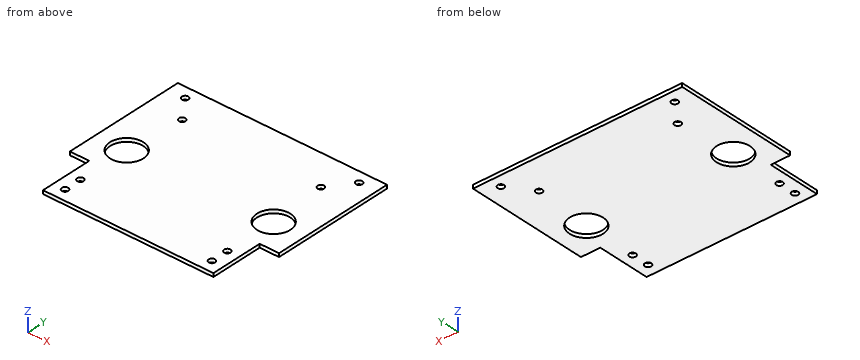
from build123d import *

# Parameters (mm, degrees)
SKETCH1_W           = 178.16
SKETCH1_H           = 150
BOSS_EXTRUDE1_DEPTH = 3
SKETCH2_R           = 14.225
SKETCH2_R_2         = 2.75
CUT_EXTRUDE1_DEPTH  = 4
SKETCH4_W           = 16.5
SKETCH4_H           = 45
CUT_EXTRUDE3_DEPTH  = 4
SKETCH5_R           = 2.75
CUT_EXTRUDE4_DEPTH  = 4


with BuildPart() as part:
    # Sketch1 → Boss-Extrude1 (new body)
    with BuildSketch(Plane.XY):
        with Locations((89.08, -75)):
            Rectangle(SKETCH1_W, SKETCH1_H)
    extrude(amount=BOSS_EXTRUDE1_DEPTH)

    # Sketch2 → Cut-Extrude1 (cut, through all)
    with BuildSketch(Plane.XY.offset(3)):
        with Locations((26.5, -80)):
            Circle(SKETCH2_R)
        with Locations((151.66, -80)):
            Circle(SKETCH2_R)
        with Locations((26.5, -140)):
            Circle(SKETCH2_R_2)
        with Locations((151.66, -140)):
            Circle(SKETCH2_R_2)
        with Locations((26.5, -125)):
            Circle(SKETCH2_R_2)
        with Locations((151.66, -125)):
            Circle(SKETCH2_R_2)
    extrude(amount=-CUT_EXTRUDE1_DEPTH, mode=Mode.SUBTRACT)

    # Sketch4 → Cut-Extrude3 (cut, through all)
    with BuildSketch(Plane.XY.offset(3)):
        with Locations((8.25, -127.5)):
            Rectangle(SKETCH4_W, SKETCH4_H)
        with Locations((169.91, -127.5)):
            Rectangle(SKETCH4_W, SKETCH4_H)
    extrude(amount=-CUT_EXTRUDE3_DEPTH, mode=Mode.SUBTRACT)

    # Sketch5 → Cut-Extrude4 (cut, through all)
    with BuildSketch(Plane.XY.offset(3)):
        with Locations((163.16, -10)):
            Circle(SKETCH5_R)
        with Locations((15, -10)):
            Circle(SKETCH5_R)
        with Locations((148.16, -30)):
            Circle(SKETCH5_R)
        with Locations((30, -30)):
            Circle(SKETCH5_R)
    extrude(amount=-CUT_EXTRUDE4_DEPTH, mode=Mode.SUBTRACT)


solid = part.part
Could you check a few things on this model? Use its own coordinates, in mm. Give positions to 0.01 mm unless a question says otherwise; leave off trailing zeros. Write each loop counter-clockwise with the first axis right and the second up, starting at its lowest first coordinate (ties: lowest second). Pieces come first, ordered by that corner, then holes. Notation, with made-up numbers: (75.25, 13) -> (125.25, 13) arc R21 ccw to (125.25, 29) -> close; hole circle Ø4 at (-31.75, 75.25). An arc over 180 degrees is marked (long way). Answer as CSV lines item,"result". Start each with the question number.
(1) If we section it at D-D, the plane y = -114: Write out the boundary of the cut face in (x, z), and give its area (3 significant figures).
(2) Please list where these lines run through material, in increasing order: line 1 (Y direction, x = 151.66, z = 2.05) (3 decimals); line 2 (Y direction, x = 15, z = 2); line 3 (Y direction, x = 24, z = 2.15).
(3) If we section it at A-A, the plane y = -30: Write out the boundary of the cut face in (x, z).
(4) I'm going to push flat-ended pins straight in: pin 1 Ø3.5 at (x, y) = (15, -10) entering from -Z; pin 2 Ø1.5 at (x, z) = (173.5, 1.5) entering from -Y. Where does each tip first touch, or does it pass through?
(5) If we section it at B-B, the plane z = 0.75: Give the number of separate pieces and of enclosed holes in the cut face, and give its area (3 significant figures).
(6) If we section it at C-C, the plane y = -80: Write out the boundary of the cut face in (x, z) (3 decimals).
Answer list:
1,outline,"(16.5, 0) -> (161.66, 0) -> (161.66, 3) -> (16.5, 3) -> close"
1,area,"435 mm^2"
2,line 1,"-150 to -142.75, -137.25 to -127.75, -122.25 to -94.225, -65.775 to 0"
2,line 2,"-105 to -88.37, -71.63 to -12.75, -7.25 to 0"
2,line 3,"-150 to -141.15, -138.85 to -126.15, -123.85 to -94, -66 to 0"
3,outline,"(0, 0) -> (27.25, 0) -> (27.25, 3) -> (0, 3) -> close; (32.75, 0) -> (145.41, 0) -> (145.41, 3) -> (32.75, 3) -> close; (150.91, 0) -> (178.16, 0) -> (178.16, 3) -> (150.91, 3) -> close"
4,pin 1,"through"
4,pin 2,"y = -105"
5,separate pieces,"1"
5,enclosed holes,"10"
5,area,"23,800 mm^2"
6,outline,"(0, 0) -> (12.275, 0) -> (12.275, 3) -> (0, 3) -> close; (40.725, 0) -> (137.435, 0) -> (137.435, 3) -> (40.725, 3) -> close; (165.885, 0) -> (178.16, 0) -> (178.16, 3) -> (165.885, 3) -> close"
